For this review, take the finished solid that the model builds, in its own axes (mm). A direction names the side the tool comes from. Round coordinates to 2 decimals unless told otherwise and drop trailing zeros. Write each loop counter-clockwise with the first axis right and the second up, starting at its lowest first coordinate (ties: lowest second). Pieces come first, ordered by that corner, then holes. Notation, with made-up numbers: (28.25, -22) - (75.25, -22) arc R6 ccw to (75.25, -15) - close; hole circle Ø6 at (-34.75, -20). An arc over 180 degrees is marked (long way). One line per item, written item: value. Start each with the question number.
Q1. Tool access review of faces 1 (the face through (-2.98, 4.68, -9.13)), 2 (the face through (-1.73, -7.81, -0.89)): name each direction out of +Z, -Z, +X, -X, +Y, -Y from which nothing blocks a thin tool from reaching the whole face with its end or side.
Q2. Clearance check with flat-ended pins moving along their axes: pin 1 Ø6 at (x, z) = (0.5, -10.5) entering from +Y; pin 2 Ø4 at (x, z) = (6, -8.5) entering from +Y; pin 3 Ø4 at (y, z) = (-4, -10.5) entering from +X. State where each tip first meets the part, or that it passes through.
Q3. Add section D-D on z = -2.5. Write out the cut boundary in (x, y), and give its area (3 significant figures).
Q4. Add section A-A on y = 0. Write out the cut boundary in (x, z), and give its area (3 significant figures).
Q5. For probe 1 along Z at (x, y) = (-3.5, 5); probe 2 along Z at (x, y) = (7, 1); probe 3 along X at (y, z) = (1.25, -6), list the stretches that pass through material, from the lowest coordinate up.
Q6. Add section C-C on z = -9. Write out the cut boundary in (x, y).
```python
from build123d import *

# Parameters (mm, degrees)
SKETCH1_R           = 8
BOSS_EXTRUDE1_DEPTH = 1.8
SKETCH2_R           = 6.5
BOSS_EXTRUDE2_DEPTH = 2.7
SKETCH3_R           = 5.55
BOSS_EXTRUDE3_DEPTH = 9.4


with BuildPart() as part:
    # Sketch1 → Boss-Extrude1 (new body)
    with BuildSketch(Plane.XY):
        Circle(SKETCH1_R)
    extrude(amount=-BOSS_EXTRUDE1_DEPTH)

    # Sketch2 → Boss-Extrude2 (add)
    with BuildSketch(Plane(origin=(0, 0, -1.8), x_dir=(-1, 0, 0), z_dir=(0, 0, -1))):
        with Locations(Location((0, 0, 0), (0, 0, 180))):
            Circle(SKETCH2_R)
    extrude(amount=BOSS_EXTRUDE2_DEPTH)

    # Sketch3 → Boss-Extrude3 (add)
    with BuildSketch(Plane(origin=(0, 0, -4.5), x_dir=(-1, 0, 0), z_dir=(0, 0, -1))):
        Circle(SKETCH3_R)
    extrude(amount=BOSS_EXTRUDE3_DEPTH)


solid = part.part
```
Result set:
1. face 1: -Z
1. face 2: +Z, -Z
2. pin 1: stops at y = 5.55
2. pin 2: stops at y = 3.85
2. pin 3: stops at x = 5.18
3. outline: circle Ø13 at (0, 0)
3. area: 133 mm^2
4. outline: (-8, -1.8) - (-6.5, -1.8) - (-6.5, -4.5) - (-5.55, -4.5) - (-5.55, -13.9) - (5.55, -13.9) - (5.55, -4.5) - (6.5, -4.5) - (6.5, -1.8) - (8, -1.8) - (8, 0) - (-8, 0) - close
4. area: 168 mm^2
5. probe 1: z = -4.5 to 0
5. probe 2: z = -1.8 to 0
5. probe 3: x = -5.41 to 5.41
6. outline: circle Ø11.1 at (0, 0)
